Source: CAD feature listing. Evaluate the final solid. Frame: model axes, mm. A direction names the side the tool comes from. Round coordinates to 2 decimals unless told otherwise and drop trailing zeros. Write each loop counter-clockwise with the first axis right and the second up, starting at its lowest first coordinate (ties: lowest second). Pieces come first, ordered by that corner, then holes. Notation, with made-up numbers: (-31.5, 29) - (3.5, 29) arc R32 cw to (3.5, 58) - close; hole circle Ø6 at (-37.5, 15.5). An arc over 180 degrees is marked (long way). Write item = value, one per line. Start each with the question number.
```python
from build123d import *

# Parameters (mm, degrees)
CROQUIS1_W              = 140
CROQUIS1_H              = 80
SALIENTE_EXTRUIR1_DEPTH = 60
CROQUIS2_R              = 17.5
SALIENTE_EXTRUIR2_DEPTH = 10
VACIADO1_T              = -2
CROQUIS3_R              = 15.5
SALIENTE_EXTRUIR3_DEPTH = 58


with BuildPart() as part:
    # Croquis1 → Saliente-Extruir1 (new body)
    with BuildSketch(Plane(origin=(0, 0, 0), x_dir=(1, 0, 0), z_dir=(0, 1, 0))):
        Rectangle(CROQUIS1_W, CROQUIS1_H)
    extrude(amount=SALIENTE_EXTRUIR1_DEPTH)

    # Croquis2 → Saliente-Extruir2 (add)
    with BuildSketch(Plane(origin=(0, 60, 0), x_dir=(1, 0, 0), z_dir=(0, 1, 0))):
        with Locations(Location((0, 0, 0), (0, 0, 270))):  # turned: the seam where the file's is
            Circle(CROQUIS2_R)
        with Locations(Location((-40, 0, 0), (0, 0, 90))):  # turned: the seam where the file's is
            Circle(CROQUIS2_R)
        with Locations(Location((40, 0, 0), (0, 0, 90))):  # turned: the seam where the file's is
            Circle(CROQUIS2_R)
    extrude(amount=SALIENTE_EXTRUIR2_DEPTH)

    # Vaciado1
    vaciado1_openings = [part.faces().sort_by_distance(p)[0] for p in [
        (0, 0, 0),
    ]]
    offset(amount=VACIADO1_T, openings=vaciado1_openings, kind=Kind.INTERSECTION)

    # Croquis3 → Saliente-Extruir3 (add)
    with BuildSketch(Plane.XZ.offset(-58)):
        with BuildLine():
            Line((-68, -2), (-19.397164741, -2))
            ThreePointArc((-19.397164741, -2), (0, -19.5), (19.397164741, -2))
            Line((19.397164741, -2), (68, -2))
            Line((68, -2), (68, 2))
            Line((68, 2), (19.397164741, 2))
            ThreePointArc((19.397164741, 2), (0, 19.5), (-19.397164741, 2))
            Line((-19.397164741, 2), (-68, 2))
            Line((-68, 2), (-68, -2))
        make_face()
        with Locations(Location((0, 0, 0), (0, 0, 270))):  # turned: the seam where the file's is
            Circle(CROQUIS3_R, mode=Mode.SUBTRACT)
    extrude(amount=SALIENTE_EXTRUIR3_DEPTH)


solid = part.part
```
(1) Contact query for a flat-ended pin moving along its axis: P1, Ø18, axis at x = -17, z = -23.5, coming from the -Y side. Output: stop coordinate, or through.
(2) Section C-C (x = 40). Return the cut outline in (y, z).
(3) Section A-A (z = 0). Return the cut outline in (x, y), plus the area to 3 significant figures.
(4) Ray query, L1, parallel to Z at x = 30, y = 26; L2, parallel to X at y = 65, z = 0; L3, parallel to Z at x = 7, y = 12.5. Return the intervals inside material, ascending. Write a range as from..to.
(5) Section D-D (z = -30.5). Return the cut outline in (x, y).
(6) Pull-direction query (X, two-part tool) for faces 1 (the flat face through (40, 70, 0)), 2 (the flat face through (70, 30, 1)), 3 (the cylindrical face through (0.401, 29.406, 19.496)); classes: +X half, -X half, draft (parallel to the pull), parting line (faces both ways), or undercut.
(7) Section B-B (y = 37). Return the cut outline in (x, z).
(8) Reachability of faces 4 (the flat face through (-1, 58, -24)), 5 (the flat face through (40, 68, 0)), 6 (the cylindrical face through (22.65, 64.93, 2.28)) from +Z, -Z, +X, -X, +Y, -Y: full face, straight path, thin tool, end or side. Return the list, or none.
Solution:
q1.P1 = 58
q2.outline = (0, -40) - (60, -40) - (60, -17.5) - (70, -17.5) - (70, 17.5) - (60, 17.5) - (60, 40) - (0, 40) - (0, 38) - (58, 38) - (58, 15.5) - (68, 15.5) - (68, -15.5) - (58, -15.5) - (58, -38) - (0, -38) - close; (0, -2) - (58, -2) - (58, 2) - (0, 2) - close
q3.outline = (-70, 0) - (-15.5, 0) - (-15.5, 68) - (15.5, 68) - (15.5, 0) - (70, 0) - (70, 60) - (57.5, 60) - (57.5, 70) - (22.5, 70) - (22.5, 60) - (17.5, 60) - (17.5, 70) - (-17.5, 70) - (-17.5, 60) - (-22.5, 60) - (-22.5, 70) - (-57.5, 70) - (-57.5, 60) - (-70, 60) - close; hole (-55.5, 58) - (-24.5, 58) - (-24.5, 68) - (-55.5, 68) - close; hole (24.5, 58) - (55.5, 58) - (55.5, 68) - (24.5, 68) - close
q3.area = 6,720 mm^2
q4.L1 = -40..-38, -2..2, 38..40
q4.L2 = -57.5..-55.5, -24.5..-22.5, -17.5..-15.5, 15.5..17.5, 22.5..24.5, 55.5..57.5
q4.L3 = -40..-38, -18.2..-13.83, 13.83..18.2, 38..40
q5.outline = (-70, 0) - (-68, 0) - (-68, 58) - (68, 58) - (68, 0) - (70, 0) - (70, 60) - (-70, 60) - close
q6.face_1 = draft
q6.face_2 = +X half
q6.face_3 = undercut
q7.outline = (-70, -40) - (70, -40) - (70, 40) - (-70, 40) - close; hole (-68, -38) - (68, -38) - (68, -2) - (19.4, -2) arc R19.5 cw to (-19.4, -2) - (-68, -2) - close; hole (-68, 2) - (-19.4, 2) arc R19.5 cw to (19.4, 2) - (68, 2) - (68, 38) - (-68, 38) - close; hole circle Ø31 at (0, 0)
q8.face_4 = -Y
q8.face_5 = none
q8.face_6 = +Y
